Input: part model. Units: mm. Frame: model coordinates. Face numbers are marked on the shaded views. A direction names the side the tool comes from. Coordinates: 2 decimals unless noted, no trailing zeros. Loops run counter-clockwise (first coordinate to the right, second up) from the corner with the lowest first, then second, coordinate; pieces in that order, holes last. Notation, with made-up numbers: (64.25, 22.25) -> (118.25, 22.25) arc R21 cw to (118.25, 61.25) -> close; hole circle Ø5 at (31.25, 26.5). An arc over 180 degrees is marked (long way). Answer as a JSON object with one key per item and string values.
from build123d import *

# Parameters (mm, degrees)
SKETCH4_R          = 7.366
CUT_EXTRUDE1_DEPTH = 12.7
SKETCH5_R          = 1.285315945
CUT_EXTRUDE2_DEPTH = 58.402876137


with BuildPart() as part:
    # Sketch3 → Revolve1 (revolve)
    with BuildSketch(Plane(origin=(0, 0, 0), x_dir=(1, 0, 0), z_dir=(0, 1, 0))):
        with BuildLine():
            Line((-13.008224719, 5.461), (-4.908764045, 5.461))
            Line((-4.908764045, 5.461), (-2.454382022, 8.763))
            Line((-2.454382022, 8.763), (2.454382022, 8.763))
            Line((2.454382022, 8.763), (2.454382022, 7.193337079))
            ThreePointArc((2.454382022, 7.193337079), (2.677566655, 6.654521711), (3.216382022, 6.431337079))
            Line((3.216382022, 6.431337079), (6.129904719, 6.431337079))
            ThreePointArc((6.129904719, 6.431337079), (6.668720086, 6.654521711), (6.891904719, 7.193337079))
            Line((6.891904719, 7.193337079), (6.891904719, 8.763))
            Line((6.891904719, 8.763), (13.18230172, 8.763))
            Line((13.18230172, 8.763), (13.18230172, 9.861582968))
            ThreePointArc((13.18230172, 9.861582968), (13.405486353, 10.400398335), (13.94430172, 10.623582968))
            Line((13.94430172, 10.623582968), (25.249181883, 10.623582968))
            Line((25.249181883, 10.623582968), (25.249181883, 11.176))
            ThreePointArc((25.249181883, 11.176), (25.472366516, 11.714815367), (26.011181883, 11.938))
            Line((26.011181883, 11.938), (32.067699775, 11.938))
            Line((32.067699775, 11.938), (32.067699775, 0))
            Line((32.067699775, 0), (-13.008224719, 0))
            Line((-13.008224719, 0), (-22.796300225, 0))
            Line((-22.796300225, 0), (-22.796300225, 2.915805843))
            Line((-22.796300225, 2.915805843), (-15.612883129, 4.357169766))
            ThreePointArc((-15.612883129, 4.357169766), (-15.538297762, 4.368329091), (-15.462974592, 4.372061052))
            Line((-15.462974592, 4.372061052), (-13.008224719, 4.372061052))
            Line((-13.008224719, 4.372061052), (-13.008224719, 5.461))
        make_face()
    revolve(axis=Axis((32.067699775, 0, 0), (-1, 0, 0)))

    # Sketch4 → Cut-Extrude1 (cut)
    with BuildSketch(Plane(origin=(32.067699775, 0, 0), x_dir=(0, 0, -1), z_dir=(1, 0, 0))):
        Circle(SKETCH4_R)
    extrude(amount=-CUT_EXTRUDE1_DEPTH, mode=Mode.SUBTRACT)

    # Sketch5 → Cut-Extrude2 (cut, through all)
    with BuildSketch(Plane.ZY.offset(22.796300225)):
        Circle(SKETCH5_R)
    extrude(amount=-CUT_EXTRUDE2_DEPTH, mode=Mode.SUBTRACT)


solid = part.part
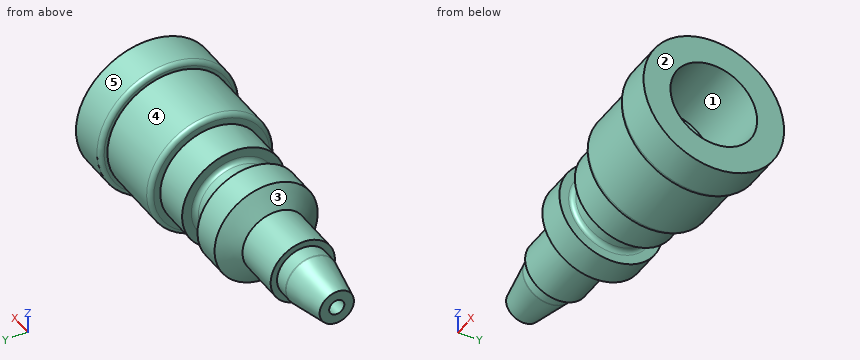
1. Mould query, pull axis Z, two halves, no side actions, for the marked faces 1, 2 and 3. Classes: pulls with the +Z half, pulls with the -Z half, needs draft (parallel to the pull), parting line crosses it, or undercut.
Reply:
{"face 1": "undercut", "face 2": "needs draft", "face 3": "parting line crosses it"}
2. Pin query (flat end, axial travel): P1, Ø4, axis at x = 23.5, z = -3, coming from the -Y side; P2, Ø8, axis at x = 3.5, z = -2, coming from the -Y side; P3, Ø6, axis at y = -4, z = -7.5, coming from the -X side; P4, Ø2, axis at x = -13.5, z = 6.5, coming from the -Y side. Return the tip coordinate at first contact, or that it passes through.
Reply:
{"P1": "stops at y = -11.41", "P2": "stops at y = -8.76", "P3": "stops at x = -4.88", "P4": "passes through"}
3. Access query for the marked faces 4 and 5. Directions: +Z, -Z, +X, -X, +Y, -Y. A direction counts if a zero-diameter tool reaches every point of the face in a straight line with its end or side. Return the directions, or none.
Reply:
{"face 4": "-X", "face 5": "+X, -X"}
4. Section query A-A (x = 10.5). Return loops of the section in (y, z).
Reply:
{"outline": "circle Ø17.53 at (0, 0); hole circle Ø2.57 at (0, 0)"}
5. Section query B-B (x = 16). Return loops of the section in (y, z), plus the area to 3 significant figures.
Reply:
{"outline": "circle Ø21.25 at (0, 0); hole circle Ø2.57 at (0, 0)", "area": "349 mm2"}
6. Line query: line 1 along Y through (x, z) = (29.25, 0); line 2 along Y through (x, z) = (-9, 0); line 3 along X through (y, z) = (-2, 4.25). Output: solid intervals per line, ascending.
Reply:
{"line 1": "y = -11.94 to -7.37, 7.37 to 11.94", "line 2": "y = -5.46 to -1.29, 1.29 to 5.46", "line 3": "x = -13.01 to 19.37"}
